Could you check a few things on this drawing? It's one solid part, dimensions in mm from its lowest x, y, z. Coordinates: 2 decimals unless noted, no trailing zeros. Write each loop counter-clockwise with the first axis right and the second up, starting at its lowest first coordinate (ties: lowest second). Pieces come first, ordered by that corner, then holes.
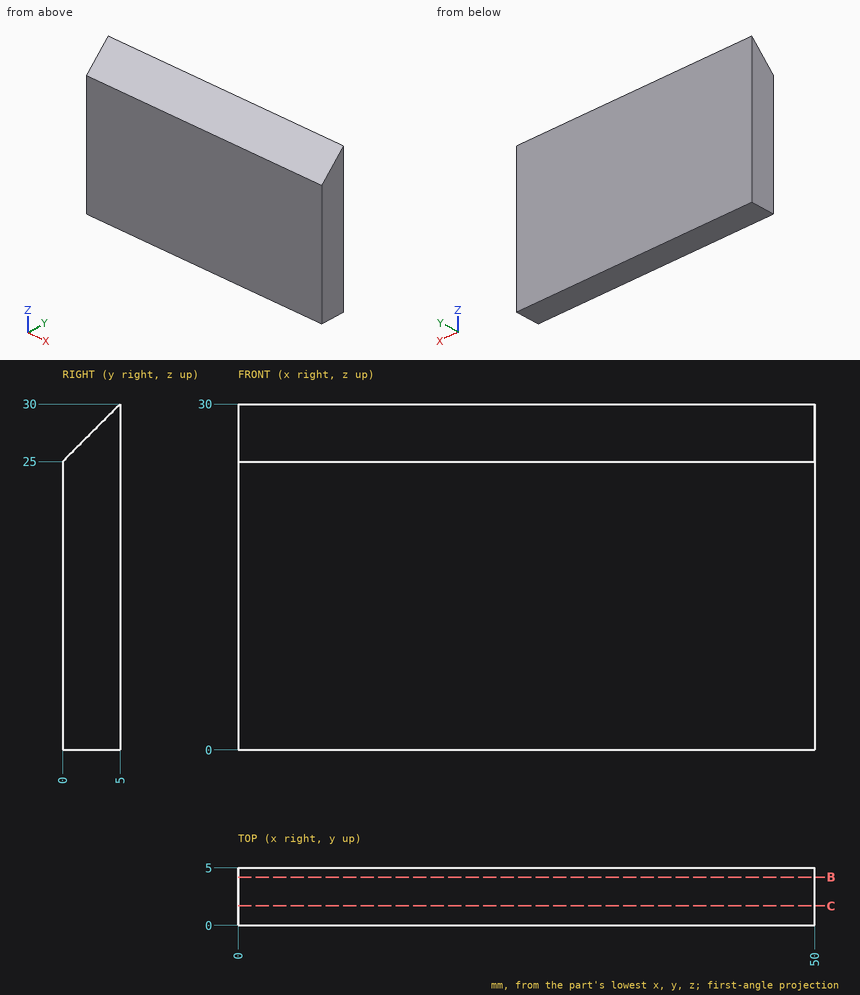
1) Imagine slicing it at B-B on y = 4.2. Please give me the cut outline in (x, z).
Values follow:
outline: (0, 0) - (50, 0) - (50, 29.2) - (0, 29.2) - close
2) I need wall thicknesses on probe 1 along Z at (x, y) = (16, 3.4); probe 2 along Z at (x, y) = (25, 4.05). Which ranges of each line are inside material? Lowest first, please.
Values follow:
probe 1: z = 0 to 28.4
probe 2: z = 0 to 29.05
3) Imagine slicing it at C-C on y = 1.7. Please give me the cut outline in (x, z), then the cut area to 4 significant figures.
Values follow:
outline: (0, 0) - (50, 0) - (50, 26.7) - (0, 26.7) - close
area: 1,335 mm2
